```python
from build123d import *

# Parameters (mm, degrees)
FRONT_START          = -3.366352234
FRONT_PLATE_DEPTH    = 2.95
CUT_EXTRUDE1_START   = 2.95
SKETCH1_W            = 3.2
SKETCH1_H            = 3.2
CUT_EXTRUDE1_DEPTH   = 12
SKETCH2_W            = 2.3
SKETCH2_H            = 5.3
CUT_EXTRUDE2_DEPTH   = 97.656428996
M3_CLEARANCE_HOLE1_D = 3.2
SKETCH5_W            = 10
SKETCH5_H            = 30
CUT_EXTRUDE3_DEPTH   = 97.656428996
FILLET1_R            = 1


# Read off the part's stored shape, not the designer's step: Front Plate
with BuildPart() as part:
    # Front Plate outline → Front Plate (new body)
    with BuildSketch(Plane.YZ.offset(FRONT_START)):
        Polygon((-23.21888173, 23.452809495), (-12.14788173, 23.452809495), (-12.14788173, 35.517809495), (-9.19788173, 35.517809495), (-9.19788173, 23.452809495), (-10.94388173, 23.452809495), (-10.94388173, 20.502809495), (-0.94388173, 20.502809495), (-0.94388173, 23.452809495), (9.05611827, 23.452809495), (9.05611827, 20.502809495), (19.05611827, 20.502809495), (19.05611827, 23.452809495), (29.05611827, 23.452809495), (29.05611827, 20.502809495), (39.05611827, 20.502809495), (39.05611827, 23.452809495), (49.05611827, 23.452809495), (49.05611827, 20.502809495), (59.05611827, 20.502809495), (59.05611827, 23.452809495), (57.31011827, 23.452809495), (57.31011827, 35.517809495), (60.26011827, 35.517809495), (60.26011827, 23.452809495), (71.33111827, 23.452809495), (71.33111827, 28.202809495), (70.28111827, 28.202809495), (70.28111827, 30.502809495), (71.33111827, 30.502809495), (71.33111827, 32.502809495), (74.53111827, 32.502809495), (74.53111827, 30.502809495), (75.58111827, 30.502809495), (75.58111827, 28.202809495), (74.53111827, 28.202809495), (74.53111827, 23.452809495), (79.05611827, 23.452809495), (79.05611827, 52.582809495), (59.05611827, 52.582809495), (59.05611827, 55.532809495), (49.05611827, 55.532809495), (49.05611827, 52.582809495), (39.05611827, 52.582809495), (39.05611827, 55.532809495), (29.05611827, 55.532809495), (29.05611827, 52.582809495), (19.05611827, 52.582809495), (19.05611827, 55.532809495), (9.05611827, 55.532809495), (9.05611827, 52.582809495), (-0.94388173, 52.582809495), (-0.94388173, 55.532809495), (-10.94388173, 55.532809495), (-10.94388173, 52.582809495), (-30.94388173, 52.582809495), (-30.94388173, 23.452809495), (-26.41888173, 23.452809495), (-26.41888173, 28.202809495), (-27.46888173, 28.202809495), (-27.46888173, 30.502809495), (-26.41888173, 30.502809495), (-26.41888173, 32.502809495), (-23.21888173, 32.502809495), (-23.21888173, 30.502809495), (-22.16888173, 30.502809495), (-22.16888173, 28.202809495), (-23.21888173, 28.202809495), align=None)
    extrude(amount=FRONT_PLATE_DEPTH)

    # Sketch1 → Cut-Extrude1 (cut)
    with BuildSketch(Plane.XY.offset(52.582809495).offset(CUT_EXTRUDE1_START)):
        with Locations((-1.891352234, 72.93111827)):
            Rectangle(SKETCH1_W, SKETCH1_H)
    cut_extrude1 = extrude(amount=-CUT_EXTRUDE1_DEPTH, mode=Mode.SUBTRACT)

    # Sketch2 → Cut-Extrude2 (cut, through all)
    with BuildSketch(Plane.ZY.offset(3.366352234)):
        with Locations((46.682809496, 72.93111827)):
            Rectangle(SKETCH2_W, SKETCH2_H)
    cut_extrude2 = extrude(amount=-CUT_EXTRUDE2_DEPTH, mode=Mode.SUBTRACT)

    # M3 Clearance Hole1 (through all)
    with Locations(Plane(origin=(-0.416352234, 0, 0), x_dir=(0, 0, -1), z_dir=(1, 0, 0))):
        with Locations((-35.517809495, 52.31011827)):
            m3_clearance_hole1 = Hole(M3_CLEARANCE_HOLE1_D / 2)

    # Mirror1: Cut-Extrude1, Cut-Extrude2, M3 Clearance Hole1 across plane
    add(cut_extrude1.mirror(Plane.ZX.offset(24.05611827)), mode=Mode.SUBTRACT)
    add(cut_extrude2.mirror(Plane.ZX.offset(24.05611827)), mode=Mode.SUBTRACT)
    add(m3_clearance_hole1.mirror(Plane.ZX.offset(24.05611827)), mode=Mode.SUBTRACT)

    # Sketch5 → Cut-Extrude3 (cut, through all)
    with BuildSketch(Plane(origin=(-0.416352234, 0, 0), x_dir=(0, 0, -1), z_dir=(1, 0, 0))):
        with Locations((-38.017809495, 24.05611827)):
            Rectangle(SKETCH5_W, SKETCH5_H)
    extrude(amount=-CUT_EXTRUDE3_DEPTH, mode=Mode.SUBTRACT)

    # Fillet1
    fillet1_edges = [part.edges().sort_by_distance(p)[0] for p in [
        (-1.891352234, 39.05611827, 33.017809495),
        (-1.891352234, 9.05611827, 33.017809495),
        (-1.891352234, 9.05611827, 43.017809495),
        (-1.891352234, 39.05611827, 43.017809495),
    ]]
    fillet(fillet1_edges, radius=FILLET1_R)


solid = part.part
```
Can you work these out from the model? Positions are in its coordinate system, mm. A direction names the side the tool comes from. Coordinates: 2 decimals unless noted, no trailing zeros. Loops run counter-clockwise (first coordinate to the right, second up) from the corner with the lowest first, then second, coordinate; pieces in that order, holes last.
1) Imagine slicing it at A-A on y = 26.5. List the corners of the cut face in (x, z) for me.
2) Imagine slicing it at D-D on x = -2.15. State how many separate pieces and enclosed holes the cut face has, plus the area to 3 significant figures.
3) Which directions (+Z, -Z, +X, -X, +Y, -Y) give clear straight access to the entire face, cutting with the end or side of a thin tool? Please do faces 4 (the flat face through (-2, -0.944, 54)), 5 (the flat face through (-2, 59.056, 22)), 6 (the flat face through (-2, 9.056, 22)).
4) Imagine slicing it at B-B on z = 49. List the corners of the cut face in (x, y) for me, plus the area to 3 significant figures.
5) Imagine slicing it at C-C on y = 7.5. List the corners of the cut face in (x, z) for me, plus the area to 3 significant figures.
6) For pin 1 (0.9 mm diameter, centred on x = -1, z = 22.5, fed in from -Y); pin 2 (0.8 mm diameter, centred on x = -2, y = -27, fed in from -Z); pin 3 (1.2 mm diameter, centred on x = -2.5, y = 75, fed in from +Z), each with a flat end and sliding along its axis, tell me the tip position at first contact or that it passes through.
7) I need wall thicknesses on probe 1 along Y at (x, z) = (-1.8, 52.5); probe 2 along Y at (x, z) = (-2.35, 23); probe 3 along Y at (x, z) = (-1.35, 30). Which ranges of each line are inside material? Lowest first, please.
8) Thinking about a two-plate mould opening in Z: for faces 1 (the flat face through (-2, 24, 43.018)), 2 (the flat face through (-2, 60.26, 30)), 3 (the flat face through (-2, -25, 32.503)), which applies, pulls with the +Z half, pulls with the -Z half, needs draft (parallel to the pull), parting line crosses it, or undercut?
Completed:
1. outline: (-3.37, 23.45) - (-0.42, 23.45) - (-0.42, 33.02) - (-3.37, 33.02) - close; (-3.37, 43.02) - (-0.42, 43.02) - (-0.42, 52.58) - (-3.37, 52.58) - close
2. separate pieces: 1
2. enclosed holes: 3
2. area: 2,920 mm2
3. face 4: +Z, +X, -X
3. face 5: -Z, +X, -X, +Y
3. face 6: -Z, +X, -X
4. outline: (-3.37, -30.94) - (-0.42, -30.94) - (-0.42, -26.42) - (-3.37, -26.42) - close; (-3.37, -23.22) - (-0.42, -23.22) - (-0.42, 71.33) - (-3.37, 71.33) - close; (-3.37, 74.53) - (-0.42, 74.53) - (-0.42, 79.06) - (-3.37, 79.06) - close
4. area: 306 mm2
5. outline: (-3.37, 23.45) - (-0.42, 23.45) - (-0.42, 52.58) - (-3.37, 52.58) - close
5. area: 85.9 mm2
6. pin 1: stops at y = -10.94
6. pin 2: stops at z = 23.45
6. pin 3: stops at z = 52.58
7. probe 1: y = -30.94 to -26.42, -23.22 to 71.33, 74.53 to 79.06
7. probe 2: y = -10.94 to -0.94, 9.06 to 19.06, 29.06 to 39.06, 49.06 to 59.06
7. probe 3: y = -30.94 to -27.47, -22.17 to -12.15, -9.2 to 57.31, 60.26 to 70.28, 75.58 to 79.06
8. face 1: undercut
8. face 2: needs draft
8. face 3: pulls with the -Z half
